Verification items for the finished model (mm, model axes). A direction names the side the tool comes from. Round coordinates to 2 decimals unless told otherwise and drop trailing zeros. Loops run counter-clockwise (first coordinate to the right, second up) from the corner with the lowest first, then second, coordinate; pieces in that order, holes last. Notation, with made-up numbers: (19, 36.25) -> (50, 36.25) arc R13 ccw to (50, 60.25) -> close; hole circle Ø10 at (18, 24.5). An arc over 180 degrees is marked (long way). Write item = value, one per line.
Autodesk Fusion 360 part; units mm, degrees
sketch "Profil" plane through (0, 0, 0) normal (0, 0, 1) x (1, 0, 0)
  circle A0 centre (0, 0) radius 4.3
  line L0 (3.8066, -2) -> (-3.8066, -2)
  line L1 (-3.8066, -2) -> (-3.8066, 2)
  line L2 (-3.8066, 2) -> (3.8066, 2)
  line L3 (3.8066, 2) -> (3.8066, -2)
  line L4 (3.8066, -2) -> (-3.8066, 2) construction
  line L5 (-3.8066, -2) -> (3.8066, 2) construction
  line L6 (2, -2) -> (-2, -2)
  line L7 (-2, -2) -> (-2, 2)
  line L8 (-2, 2) -> (2, 2)
  line L9 (2, 2) -> (2, -2)
  line L10 (2, -2) -> (-2, 2) construction
  line L11 (-2, -2) -> (2, 2) construction
  line L12 (3.6946, 2.2) -> (3.6946, -2.2)
  dimension "d1" = 8.6
  dimension "d2" = 4
  dimension "d3" = 4
  dimension "d4" = 0.2
extrude "Extrude1" add sketch "Profil" along normal blind 88.5 contours A0 L2 L8 L12 | A0 L0 L6 L12 | L0 L2 L6 L7 L8 L9
fillet "Fillet1" radius 0.1 2 edges at (-3.8066, 2, 44.25) (-3.8066, -2, 44.25)
chamfer "Chamfer1" distance 0.1 angle 45 4 edges at (-2, -2, 44.25) (-2, 2, 44.25) (2, -2, 44.25) (2, 2, 44.25)
chamfer "Chamfer2" distance 0.1 angle 45 2 faces at (0.6667, -0.6333, 88.5) (0.6667, -0.6333, 0)
(1) Set-up check for faces 1 (the face through (0, 0, 0)), 2 (the face through (3, -2, 44)), 3 (the face through (-3, -2, 44)): record each of +Z, -Z, +X, -X, +Y, -Y from which the full face is reachable in a straight line by a thin tool's end or side.
Filled sheet:
face_1 = -Z, +X, -X, +Y, -Y
face_2 = +Z, -Z, +X
face_3 = +Z, -Z, -X
(2) Go/stop test with flat-tipped pins: pin 1 Ø0.8 at (x, z) = (-2.5, 25) entering from -Y; pin 2 Ø4 at (y, z) = (0.5, 31) entering from +X; pin 3 Ø1.1 at (y, z) = (-0.5, 45.5) entering from -X; pin 4 Ø0.5 at (x, z) = (-3, 66) entering from +Y. Record where each tip stops, or that it passes through.
Filled sheet:
pin_1 = -3.75
pin_2 = 3.69
pin_3 = -2
pin_4 = 3.31
(3) Draft check along Y on faces 4 (the face through (3, 2, 44)), 5 (the face through (0, -4.3, 43.6)), 6 (the face through (-0.1, 4.3, 43.6)). Enter one of: released by +Y, released by -Y, zero draft, split by the parting line, or undercut.
Filled sheet:
face_4 = undercut
face_5 = released by -Y
face_6 = released by +Y
(4) Sectioned sample at B-B, the plane z = 13. Record the cut outline in (x, y).
Filled sheet:
outline = (-3.72, -2.15) arc R4.3 ccw to (3.69, -2.2) -> (3.69, -2) -> (2.1, -2) -> (2, -1.9) -> (2, 1.9) -> (2.1, 2) -> (3.69, 2) -> (3.69, 2.2) arc R4.3 ccw to (-3.72, 2.15) arc R0.1 ccw to (-3.64, 2) -> (-2.1, 2) -> (-2, 1.9) -> (-2, -1.9) -> (-2.1, -2) -> (-3.64, -2) arc R0.1 ccw to start
(5) Material ranges on probe 1 along X at (y, z) = (3.75, 60.5); probe 2 along Y at (x, z) = (3.5, 9); probe 3 along Y at (x, z) = (2.5, 71.5), recorded low to high. Write a range as from..to.
Filled sheet:
probe_1 = -2.1..2.1
probe_2 = -2.5..-2, 2..2.5
probe_3 = -3.5..-2, 2..3.5
(6) Sectioned sample at A-A, the plane y = -1. Record the cut outline in (x, z), and give its area (3 significant figures).
Filled sheet:
outline = (-2, 0.1) -> (-1.9, 0) -> (1.9, 0) -> (2, 0.1) -> (2, 88.4) -> (1.9, 88.5) -> (-1.9, 88.5) -> (-2, 88.4) -> close
area = 354 mm2
